Job drawing, mm, ordinate dimensions from the low corner. One solid piece. Coordinates: 2 decimals unless noted, no trailing zeros. Write each loop counter-clockwise with the first axis right and the second up, starting at its lowest first coordinate (ties: lowest second). Pieces come first, ordered by that corner, then holes. Notation, with made-up numbers: (61, 69) -> (66, 69) arc R12 ccw to (66, 74) -> close; hole circle Ø9 at (6, 74). An arc over 180 degrees is marked (long way). One line per question, with ' | ' between items. Start each with the question number.
Item 1: Saw through at B-B (z = 28). List the corners of the cut face in (x, y).
Item 2: Saw through at D-D (x = 8). List the corners of the cut face in (y, z), and give its area (3 significant figures).
Item 3: Pin check, flat tip, straight feed: pin 1 (1 mm diameter, centred on x = 8, y = 1.5, fed in from -Z). Stop position of the tip, or through.
Item 4: Saw through at C-C (y = 0.5). Count the separate pieces of the cut face and the enclosed holes in it, and give its area (3 significant figures).
Item 5: Saw through at A-A (x = 28). List the corners of the cut face in (y, z).
Item 6: Probe probe 1 along X at (y, z) = (1.4, 48); probe 2 along Z at (x, y) = (28, 1.2); probe 3 along X at (y, z) = (1.6, 8). List the from-to ranges inside material, lowest first. Write a range as [from, to].
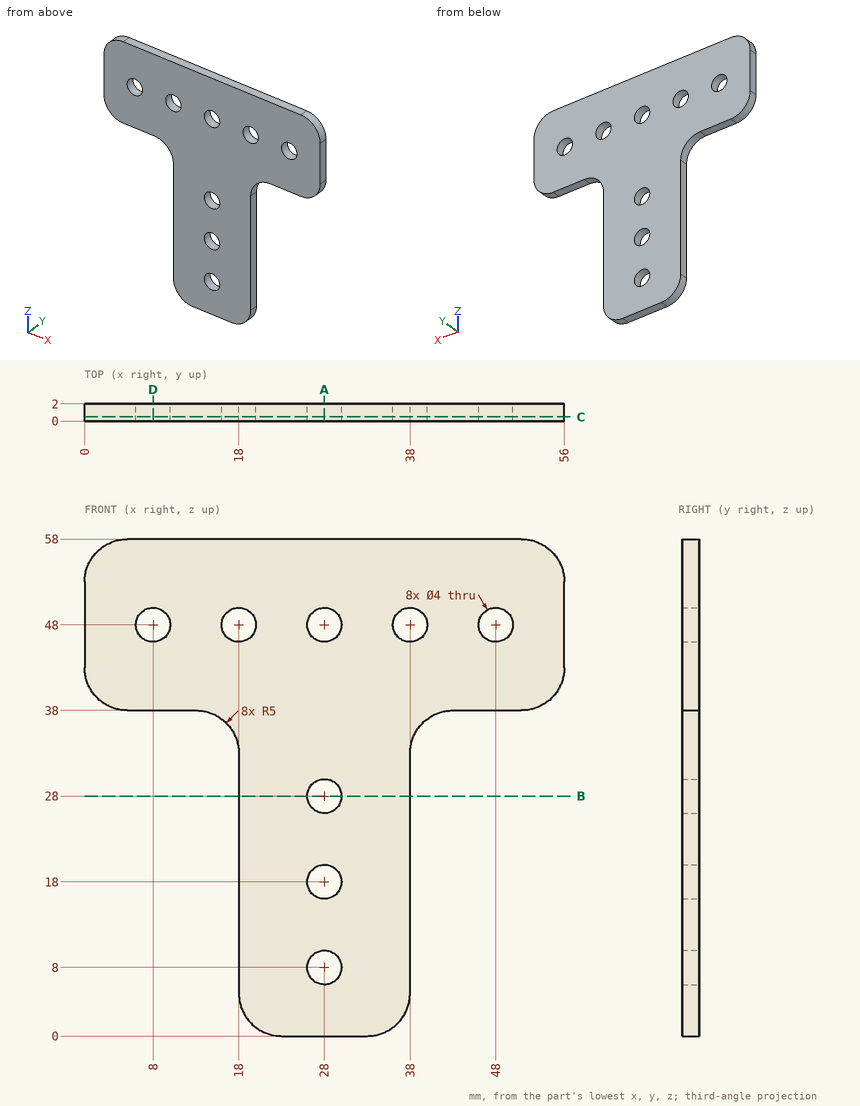
From the geometry:
1) outline: (18, 0) -> (26, 0) -> (26, 2) -> (18, 2) -> close; (30, 0) -> (38, 0) -> (38, 2) -> (30, 2) -> close
2) outline: (0, 38) -> (2, 38) -> (2, 46) -> (0, 46) -> close; (0, 50) -> (2, 50) -> (2, 58) -> (0, 58) -> close | area: 32.0 mm2
3) pin 1: z = 38
4) separate pieces: 1 | enclosed holes: 8 | area: 1,760 mm2
5) outline: (0, 0) -> (2, 0) -> (2, 6) -> (0, 6) -> close; (0, 10) -> (2, 10) -> (2, 16) -> (0, 16) -> close; (0, 20) -> (2, 20) -> (2, 26) -> (0, 26) -> close; (0, 30) -> (2, 30) -> (2, 46) -> (0, 46) -> close; (0, 50) -> (2, 50) -> (2, 58) -> (0, 58) -> close
6) probe 1: [0, 6], [10, 16], [20, 26], [30, 36], [40, 46], [50, 56] | probe 2: [0, 6], [10, 16], [20, 26], [30, 46], [50, 58] | probe 3: [18, 26], [30, 38]
